Geometry: final body of the model. Coordinates: model frame, mm. Give positions to 0.01 mm unless a question says otherwise; leave off trailing zeros. Order: outer loops, then holes, each group sorted by start corner. A loop starts at its lowest first (then second) coordinate and runs counter-clockwise, first axis right, second up. Notation, with made-up numbers: M -3,36.25 L 3,36.25 A31 ccw 3,64.25 Z; hole C -19,63.25 d9. An arc over 180 degrees is marked long. Use CSV: the item, a comma, the result in double quotes.
Autodesk Inventor part; units mm, degrees
ref_plane "YZ Plane" through (0, 0, 0) normal (1, 0, 0) x (0, 1, 0)
ref_plane "XZ Plane" through (0, 0, 0) normal (0, 1, 0) x (-1, 0, 0)
ref_plane "XY Plane" through (0, 0, 0) normal (0, 0, 1) x (1, 0, 0)
sketch "Absorber-Base" plane through (0, 0, 0) normal (0, 0, 1) x (1, 0, 0)
  line L0 (-19.0625, 19.0625) -> (19.0625, 19.0625)
  line L1 (19.0625, 19.0625) -> (19.0625, -19.0625)
  line L2 (19.0625, -19.0625) -> (-19.0625, -19.0625)
  line L3 (-19.0625, -19.0625) -> (-19.0625, 19.0625)
  line L4 (-19.0625, 19.0625) -> (19.0625, -19.0625) construction
  line L5 (19.0625, 19.0625) -> (-19.0625, -19.0625) construction
  point P0 (0, 0)
  dimension "d0" = 38.125
extrude "Gesamtvolumen" add sketch "Absorber-Base" along normal blind 115
sketch "Skizze2" plane through (0, 0, 0) normal (0, 1, 0) x (-1, 0, 0)
  line L0 (-28, 0) -> (28, 0)
  line L1 (19.0625, 0) -> (19.0625, 115)
  line L2 (-19.0625, 0) -> (-19.0625, 115)
  line L3 (19.0625, 0) -> (-19.0625, 0)
  line L4 (-19.0625, 0) -> (-19.0625, 10)
  line L5 (-19.0625, 10) -> (19.0625, 10)
  line L6 (19.0625, 10) -> (19.0625, 0)
  line L7 (-19.0625, 115) -> (19.0625, 115)
  line L8 (0, 115) -> (19.0625, 10)
  line L9 (0, 115) -> (-19.0625, 10)
  point P0 (0, 0)
  point P1 (19.0625, 10)
  dimension "d6" = 10
extrude "Cutaway" cut sketch "Skizze2" along normal mid plane 38.125 contours L2 L7 L9 | L8 L7 L1
pattern_circular "Runde Anordnung1" count 2 over 90 about axis through (0, 0, -10) along (0, 0, 1) of "Cutaway"
equation "\"d0\" = Base_Seitenlänge"
equation "\"d1\" = Gesamthöhe"
equation "\"d6\" = Base_Höhe"
equation "\"d7\" = Base_Seitenlänge"
equation "\"Base_Seitenlänge\" = 38.125"
equation "\"Base_Höhe\" = 10"
equation "\"Gesamthöhe\" = 115"
properties part number "HF-Absorber-dummy"
1. Line query: line 1 (Y direction, x = -10.5, z = 40); line 2 (X direction, y = -4, z = 28); line 3 (Y direction, x = -2, z = 23). Output: solid intervals per line, ascending.
Answer:
line 1,"-13.62 to 13.62"
line 2,"-15.79 to 15.79"
line 3,"-16.7 to 16.7"
2. Section B-B, the plane x = -8. Return the cut outline in (y, z), plus the area to 3 significant figures.
Answer:
outline,"M -19.06,0 L 19.06,0 L 19.06,10 L 8,70.93 L -8,70.93 L -19.06,10 Z"
area,"2,030 mm2"
3. Section C-C, the plane z = 28.5. Return the cut outline in (x, y), plus the area to 3 significant figures.
Answer:
outline,"M -15.7,-15.7 L 15.7,-15.7 L 15.7,15.7 L -15.7,15.7 Z"
area,"986 mm2"
4. Section A-A, the plane y = -4.5. Return the cut outline in (x, z), plus the area to 3 significant figures.
Answer:
outline,"M -19.06,0 L 19.06,0 L 19.06,10 L 4.5,90.21 L -4.5,90.21 L -19.06,10 Z"
area,"2,270 mm2"
5. Section D-D, the plane z = 51. Return the cut outline in (x, y).
Answer:
outline,"M -11.62,-11.62 L 11.62,-11.62 L 11.62,11.62 L -11.62,11.62 Z"
6. Pin query (flat end, axial travel): pin 1 Ø4 at (y, z) = (5.5, 55) entering from +X; pin 2 Ø3 at (y, z) = (5.5, 49) entering from +X; pin 3 Ø10 at (x, z) = (13, 48.5) entering from -Y. Return the tip coordinate at first contact, or that it passes through.
Answer:
pin 1,"x = 11.26"
pin 2,"x = 12.25"
pin 3,"y = -12.98"
